Autodesk Inventor part; units mm, degrees
ref_plane "YZ Plane" through (0, 0, 0) normal (1, 0, 0) x (0, 1, 0)
ref_plane "XZ Plane" through (0, 0, 0) normal (0, 1, 0) x (-1, 0, 0)
ref_plane "XY Plane" through (0, 0, 0) normal (0, 0, 1) x (1, 0, 0)
sketch "Sketch1" plane through (0, 0, 0) normal (0, 1, 0) x (-1, 0, 0)
  arc A0 (-1.55, 0) -> (-0.0788, 1.548) centre (0, 0) ccw
  line L0 (-1.55, 14.25) -> (-1.55, 0)
  arc A1 (-1.55, 2.9462) -> (-0.0788, 1.548) centre (-0.15, 2.9462) ccw
  arc A2 (-0.35, 3.0996) -> (0.0435, 2.6996) centre (0.05, 3.0996) ccw
  line L1 (-1.55, 14.25) -> (-0.35, 14.25)
  line L2 (-0.35, 14.25) -> (-0.35, 3.0996)
  line L3 (-2.7, 14.25) -> (-2.7, 0)
  line L4 (-2.7, 14.25) -> (-1.55, 14.25)
  arc A3 (-2.7, 0) -> (0.0435, 2.6996) centre (0, 0) ccw
  dimension "d0" = 3.1
  dimension "d1" = 2.8
  dimension "d2" = 14.25
  dimension "d6" = 0.8
extrude "Extrusion1" add sketch "Sketch1" along normal blind 9.8
sketch "Sketch2" plane through (0.35, 0, 3.0996) normal (-1, 0, 0) x (0, 0, 1)
  line L0 (6.0004, -8.6055) -> (6.0004, 17.2383) construction
  line L1 (-11.7051, 4.9) -> (18.5644, 4.9) construction
  line L2 (11.1504, 0) -> (11.1504, 9.8) construction
  line L3 (-3.0996, 0) -> (-0.3999, 0) construction
  line L4 (-0.3999, 0) -> (-0.3999, 9.8) construction
  line L5 (-3.0996, 9.8) -> (-0.3999, 9.8) construction
  line L6 (-3.0996, 0) -> (-3.0996, 9.8) construction
  line L7 (-3.0996, 0) -> (-3.0996, 9.8) construction
  line L8 (-5.7996, 0) -> (-5.7996, 9.8) construction
  point P0 (11.1504, 4.9)
  point P1 (6.0004, 4.9)
  dimension "d9" = 11.8
hole "Hole1" at (0.35, 4.9, 9.1) direction (1, 0, 0) diameter 4.8 end through all
fillet "Fillet1" radius 4.8 2 edges at (1.525, 9.8, 14.25) (1.525, 0, 14.25)
properties part number "Cable Clip 3-1Dia RS817-8956"
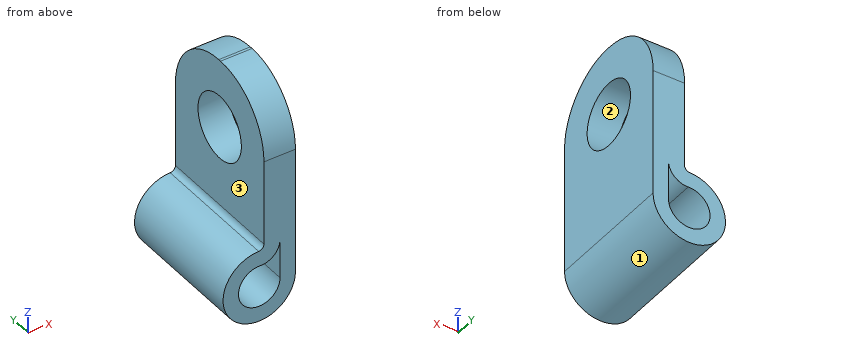
Here's how the part is built. I have some questions about the finished solid (model axes, mm). Face numbers are marked on the shaded views. Give positions to 0.01 mm unless a question says otherwise; leave off trailing zeros. Write each loop counter-clockwise with the first axis right and the second up, starting at its lowest first coordinate (ties: lowest second). Pieces come first, ordered by that corner, then holes.
(1) Thinking about a two-plate mould opening in Z: for the marked faces 1, 2 and 3, which applies, pulls with the +Z half, pulls with the -Z half, needs draft (parallel to the pull), parting line crosses it, or undercut?
Output values:
face 1: parting line crosses it
face 2: undercut
face 3: needs draft
(2) Imagine slicing it at C-C, the plane x = -0.3. Write out the boundary of the cut face in (y, z), and give its area (3 significant figures).
Output values:
outline: (0, -2.68) - (9.8, -2.68) - (9.8, -1.52) - (0, -1.52) - close; (0, 1.52) - (9.8, 1.52) - (9.8, 2.68) - (0, 2.68) - close
area: 22.8 mm2
(3) Imagine slicing it at B-B, the plane y = 3.5. Write out the boundary of the cut face in (x, z).
Output values:
outline: (-0.04, 2.7) arc R2.7 ccw (long way) to (2.7, 0) - (2.7, 7.15) - (0.35, 7.15) - (0.35, 3.1) arc R0.4 cw to start; (0.35, 11.05) - (2.7, 11.05) - (2.7, 14.07) - (0.35, 14.07) - close; hole (0.08, 1.55) arc R1.55 ccw (long way) to (1.55, 0) - (1.55, 2.95) arc R1.4 cw to start
(4) If I drill on L1, parallel to Z at x = 1.3, y = 4.75; L2, parallel to Y at x = 1.85, z = 9.1; L3, parallel to X at y = 7.25, z = 5.5, over which ranges is the centre line in solid material (lowest first)?
Output values:
L1: z = -2.37 to -0.84, 2.15 to 6.7, 11.5 to 14.25
L2: y = 0 to 2.5, 7.3 to 9.8
L3: x = 0.35 to 2.7
(5) Will these pins go through, and if not, where does the flat tip stop? pin 1 (3 mm diameter, centred on y = 4.9, z = 9.1, fed in from -X); pin 2 (3 mm diameter, centred on y = 6.5, z = 7, fed in from -X).
Output values:
pin 1: passes through
pin 2: stops at x = 0.35
(6) Imagine slicing it at A-A, the plane z = 9.1. Write out the boundary of the cut face in (x, y), and give its area (4 significant figures).
Output values:
outline: (0.35, 0) - (2.7, 0) - (2.7, 2.5) - (0.35, 2.5) - close; (0.35, 7.3) - (2.7, 7.3) - (2.7, 9.8) - (0.35, 9.8) - close
area: 11.75 mm2
(7) Imagine slicing it at D-D, the plane y = 7.5. Write out the boundary of the cut face in (x, z).
Output values:
outline: (-0.04, 2.7) arc R2.7 ccw (long way) to (2.7, 0) - (2.7, 13.55) - (0.35, 13.55) - (0.35, 3.1) arc R0.4 cw to start; hole (0.08, 1.55) arc R1.55 ccw (long way) to (1.55, 0) - (1.55, 2.95) arc R1.4 cw to start
